Source: CAD feature listing. Evaluate the final solid. Frame: model axes, mm. A direction names the side the tool comes from. Give positions to 0.01 mm unless a question says otherwise; leave off trailing zeros. Loops run counter-clockwise (first coordinate to the right, second up) from the corner with the lowest first, then second, coordinate; pieces in that order, holes last. Notation, with made-up numbers: (11, 41.25) - (57, 41.25) arc R16 cw to (57, 54.25) - close; hole circle Ø5 at (86.25, -37). An arc over 180 degrees is marked (long way). Write each question's results on one line, items separated by ' | '. Start each with the question number.
(1) Material intervals for line 1 along X through (y, z) = (8.75, 3.5) (3 decimals); line 2 along Z through (x, y) = (0.5, -8.75); line 3 along Y through (x, z) = (-4.75, 1.5) (3 decimals), sorted ascending. Write a range as [from, to].
(2) Contact query for flat-ended pins moving along their axis: pin 1 (3 mm diameter, centred on x = 1, y = 3.5, fed in from +Z); pin 2 (1.2 mm diameter, centred on x = -10, z = 7.5, fed in from -Y); pin 3 (0.9 mm diameter, centred on x = -10, z = 6.5, fed in from +Y). Output: stop coordinate, or through.
(3) Cut plane C-C on z = 1.5. Return the cut outline in (x, y) (3 decimals), then the cut area to 3 significant figures.
(4) Pull-direction query (X, two-part tool) for faces 6 (the flat face through (-7.75, -12.4, 4.5)), 7 (the flat face through (9.5, 11.7, 5.6)), 8 (the flat face through (10.2, 0, 3)); classes: pulls with the +X half, pulls with the -X half, needs draft (parallel to the pull), parting line crosses it, or undercut.
(5) Cut plane B-B on y = 9.25. Return the cut outline in (x, z) (3 decimals), then the cut area to 4 significant figures.
(6) Reachability of faces 1 (the flat face through (-10, 10.9, 7)), 2 (the flat face through (-9.075, 0, 4)), 3 (the flat face through (10, 8.1, 7)), 4 (the flat face through (9.7, -12.5, 2.8)), 5 (the flat face through (-6.25, -12.4, 4.6)) from +Z, -Z, +X, -X, +Y, -Y: full face, straight path, thin tool, end or side. Return the list, or none.
(7) Cut plane D-D on x = -3.5. Return the cut outline in (y, z) (3 decimals).
(8) Cut plane A-A on z = 7. Return the cut outline in (x, y) (3 decimals).
from build123d import *

# Parameters (mm, degrees)
SKETCH11_W          = 20.4
SKETCH11_H          = 26
BOSS_EXTRUDE5_DEPTH = 1
BOSS_EXTRUDE6_DEPTH = 4.6
CHAMFER2_SIZE       = 1
CUT_EXTRUDE1_REACH  = 30.485
SKETCH14_W          = 1.125
SKETCH14_H          = 2.8
BOSS_EXTRUDE7_DEPTH = 2.4


with BuildPart() as part:
    # Sketch11 → Boss-Extrude5 (new body)
    with BuildSketch(Plane.XY):
        Rectangle(SKETCH11_W, SKETCH11_H)
    extrude(amount=BOSS_EXTRUDE5_DEPTH)

    # Sketch12 → Boss-Extrude6 (add)
    with BuildSketch(Plane.XY.offset(1)):
        Polygon((-10.2, 13), (-10.2, -13), (10.2, -13), (10.2, 13), (9.075, 13), (9.075, -11.875), (-9.075, -11.875), (-9.075, 13), align=None)
    extrude(amount=BOSS_EXTRUDE6_DEPTH)

    # Chamfer2
    chamfer2_edges = [part.edges().sort_by_distance(p)[0] for p in [
        (-10.2, 13, 2.8),
        (10.2, 13, 2.8),
        (10.2, -13, 2.8),
        (-10.2, -13, 2.8),
    ]]
    chamfer(chamfer2_edges, length=CHAMFER2_SIZE)

    # Sketch13 → Cut-Extrude1 (cut, up to next)
    with BuildSketch(Plane.XZ.offset(13), mode=Mode.PRIVATE) as cut_extrude1_sk1:
        with BuildLine():
            Line((-7.75, 5.6), (-6.25, 5.6))
            Line((-6.25, 5.6), (-6.25, 3.5))
            ThreePointArc((-6.25, 3.5), (-7, 2.75), (-7.75, 3.5))
            Line((-7.75, 3.5), (-7.75, 5.6))
        make_face()
    cut_extrude1_tool1 = extrude(cut_extrude1_sk1.sketch, amount=-CUT_EXTRUDE1_REACH, mode=Mode.PRIVATE) & part.part
    # Sketch13 → Cut-Extrude1 (cut, up to next)
    with BuildSketch(Plane.XZ.offset(13), mode=Mode.PRIVATE) as cut_extrude1_sk2:
        with BuildLine():
            Line((7.75, 5.6), (4.75, 5.6))
            Line((4.75, 5.6), (4.75, 3.5))
            ThreePointArc((4.75, 3.5), (4.969669914, 2.969669914), (5.5, 2.75))
            Line((5.5, 2.75), (7, 2.75))
            ThreePointArc((7, 2.75), (7.530330086, 2.969669914), (7.75, 3.5))
            Line((7.75, 3.5), (7.75, 5.6))
        make_face()
    cut_extrude1_tool2 = extrude(cut_extrude1_sk2.sketch, amount=-CUT_EXTRUDE1_REACH, mode=Mode.PRIVATE) & part.part
    add(cut_extrude1_tool1.solids().sort_by_distance((-7, -13, 4.250265))[0], mode=Mode.SUBTRACT)
    add(cut_extrude1_tool2.solids().sort_by_distance((6.25, -13, 4.211539))[0], mode=Mode.SUBTRACT)

    # Sketch14 → Boss-Extrude7 (add)
    with BuildSketch(Plane.XY.offset(5.6)):
        with Locations((-9.6375, 9.5)):
            Rectangle(SKETCH14_W, SKETCH14_H)
        with Locations((9.6375, 9.5)):
            Rectangle(SKETCH14_W, SKETCH14_H)
    extrude(amount=BOSS_EXTRUDE7_DEPTH)


solid = part.part
Ans:
1) line 1: [-10.2, -9.075], [9.075, 10.2] | line 2: [0, 1] | line 3: [-13, -11.875]
2) pin 1: z = 1 | pin 2: y = 8.1 | pin 3: y = 10.9
3) outline: (-10.2, -12) - (-9.2, -13) - (9.2, -13) - (10.2, -12) - (10.2, 12) - (9.2, 13) - (9.075, 13) - (9.075, -11.875) - (-9.075, -11.875) - (-9.075, 13) - (-9.2, 13) - (-10.2, 12) - close | area: 76.9 mm^2
4) face 6: undercut | face 7: needs draft | face 8: pulls with the +X half
5) outline: (-10.2, 0) - (10.2, 0) - (10.2, 8) - (9.075, 8) - (9.075, 1) - (-9.075, 1) - (-9.075, 8) - (-10.2, 8) - close | area: 36.15 mm^2
6) face 1: +Z, +X, -X, +Y | face 2: +Z, +Y | face 3: +Z, +X, -X, -Y | face 4: +Z, -Z, +X, -Y | face 5: +Z, +Y, -Y
7) outline: (-13, 0) - (13, 0) - (13, 1) - (-11.875, 1) - (-11.875, 5.6) - (-13, 5.6) - close
8) outline: (-10.2, 8.1) - (-9.075, 8.1) - (-9.075, 10.9) - (-10.2, 10.9) - close; (9.075, 8.1) - (10.2, 8.1) - (10.2, 10.9) - (9.075, 10.9) - close
